Autodesk Inventor part; units mm, degrees
ref_plane "YZ Plane" through (0, 0, 0) normal (1, 0, 0) x (0, 1, 0)
ref_plane "XZ Plane" through (0, 0, 0) normal (0, 1, 0) x (-1, 0, 0)
ref_plane "XY Plane" through (0, 0, 0) normal (0, 0, 1) x (1, 0, 0)
sketch "Sketch1" plane through (0, 0, 0) normal (0, 0, 1) x (1, 0, 0)
  line L0 (0, 0) -> (0, 13)
  line L1 (0, 13) -> (22.5, 13)
  line L2 (22.5, 13) -> (24.5, 13)
  line L3 (24.5, 13) -> (24.5, 7)
  line L4 (24.5, 7) -> (22.5, 7)
  line L5 (22.5, 7) -> (22.5, 0)
  line L6 (22.5, 0) -> (0, 0)
  dimension "d0" = 13
  dimension "d3" = 22.5
  dimension "d4" = 2
  dimension "d5" = 6
  dimension "d6" = 2
  dimension "d7" = 7
revolve "Revolution1" add sketch "Sketch1" angle 360 about axis through (0, 0, 0) along (0, 1, 0)
sketch "Sketch2" plane through (0, 13, 0) normal (0, 1, 0) x (1, 0, 0)
  line L0 (0.75, 13) -> (-0.75, 13)
  line L1 (-0.75, 13) -> (-0.75, -13)
  line L2 (-0.75, -13) -> (0.75, -13)
  line L3 (0.75, -13) -> (0.75, 13)
  point P0 (0, 0)
  dimension "d9" = 1.5
  dimension "d10" = 26
  dimension "d11" = 13
  dimension "d12" = 0.75
extrude "Extrusion1" cut sketch "Sketch2" against normal through all
fillet "Fillet1" radius 6 4 edges at (-0.75, 13, 0) (0.75, 13, 0) (-0.75, 0, 0) (0.75, 0, 0)
chamfer "Chamfer1" distance 4 angle 45 1 edges at (-24.5, 13, 0)
fillet "Fillet2" radius 0.5 4 edges at (0, 13, -13) (0, 13, 13) (0, 0, -13) (0, 0, 13)
properties part number "head_innter_top" material "Aluminum 6061"
The model under review builds one solid part; all positions refer to its coordinate system, in mm. A direction names the side the tool comes from. Coordinates: 2 decimals unless noted, no trailing zeros. Write each loop counter-clockwise with the first axis right and the second up, starting at its lowest first coordinate (ties: lowest second). Pieces come first, ordered by that corner, then holes.
1) We need section A-A on x = 0. State the section outline as (y, z) points, then the cut area to 3 significant figures.
2) We need section D-D on y = 11.25. State the section outline as (x, z) points.
3) To check wall thickness, follow probe 1 along X at (y, z) = (8, -7.5); probe 2 along X at (y, z) = (8.25, 11); probe 3 along Z at (x, y) = (1, 5.25). State the ranges of each line that lie inside material, in increasing order.
4) Machinability: for faces 1 (the face through (11, 7, 20)), 2 (the face through (-2.461, 11.196, 0.189)), 3 (the face through (13.17, 7.99, 20.66)), 4 (the face through (0, 7, 13)), which of the approach directions +Z, -Z, +X, -X, +Y, -Y give a long, thin tool a straight path to every point of the face, cutting with its end or side? Answer none if there is none.
5) Clearance check with flat-ended pins moving along their axes: pin 1 Ø0.5 at (y, z) = (6.5, -5.5) entering from -X; pin 2 Ø6 at (x, y) = (12, 2) entering from -Z; pin 3 Ø1.1 at (y, z) = (6.5, 5.5) entering from +X; pin 4 Ø10 at (x, z) = (-7, 9) entering from -Y. State where each tip first meets the part, or that it passes through.
6) We need section B-B on z = 0. State the section outline as (x, y) points.
7) We need section C-C on y = 1.75. State the section outline as (x, z) points, then the cut area to 3 significant figures.
8) The part is to be moulded in two halves that separate along Z. For faces 5 (the face through (10.382, 3.451, -19.961)), 6 (the face through (2.554, 1.711, -0.189)), 7 (the face through (10, 0, 0)), say which applies: pulls with the +Z half, pulls with the -Z half, needs draft (parallel to the pull), parting line crosses it, or undercut.
Answer list:
1. outline: (0, -22.5) - (7, -22.5) - (7, -24.5) - (9, -24.5) - (13, -20.5) - (13, -13.5) arc R0.5 ccw to (12.5, -13) - (0.5, -13) arc R0.5 ccw to (0, -13.5) - close; (0, 13.5) arc R0.5 ccw to (0.5, 13) - (12.5, 13) arc R0.5 ccw to (13, 13.5) - (13, 20.5) - (9, 24.5) - (7, 24.5) - (7, 22.5) - (0, 22.5) - close
1. area: 255 mm2
2. outline: circle Ø44.5 at (0, 0); hole (-2.51, -13) - (2.51, -13) - (2.51, 13) - (-2.51, 13) - close
3. probe 1: x = -23.32 to -0.83, 0.83 to 23.32
3. probe 2: x = -21.89 to -0.88, 0.88 to 21.89
3. probe 3: z = -22.48 to 22.48
4. face 1: -Y
4. face 2: +Y
4. face 3: +Y, -Y
4. face 4: none
5. pin 1: stops at x = -21.88
5. pin 2: stops at z = -20.62
5. pin 3: stops at x = 23.93
5. pin 4: stops at y = 0
6. outline: (-24.5, 7) - (-22.5, 7) - (-22.5, 0) - (-6.75, 0) arc R6 ccw to (-0.75, 6) - (-0.75, 7) arc R6 ccw to (-6.75, 13) - (-20.5, 13) - (-24.5, 9) - close; (0.75, 6) arc R6 ccw to (6.75, 0) - (22.5, 0) - (22.5, 7) - (24.5, 7) - (24.5, 9) - (20.5, 13) - (6.75, 13) arc R6 ccw to (0.75, 7) - close
7. outline: circle Ø45 at (0, 0); hole (-2.51, -13) - (2.51, -13) - (2.51, 13) - (-2.51, 13) - close
7. area: 1,460 mm2
8. face 5: parting line crosses it
8. face 6: undercut
8. face 7: needs draft
